from build123d import *

# Parameters (mm, degrees)
SKETCH1_R           = 1.7018
BOSS_EXTRUDE1_DEPTH = 2.5019
BOSS_EXTRUDE2_DEPTH = 4.5339
SKETCH3_R           = 2.032
BOSS_EXTRUDE3_DEPTH = 0.8128
SKETCH4_R           = 1.77918252
BOSS_EXTRUDE4_DEPTH = 1.0033


with BuildPart() as part:
    # Sketch1 → Boss-Extrude1 (new body)
    with BuildSketch(Plane(origin=(0, 0, 0), x_dir=(1, 0, 0), z_dir=(0, 1, 0))):
        with BuildLine():
            Line((27.1272, -31.8389), (27.1272, -19.9898))
            Line((27.1272, -19.9898), (25.072658108, -8.860571344))
            ThreePointArc((25.072658108, -8.860571344), (22.793680926, -7.133528849), (20.8661, -9.2456))
            Line((20.8661, -9.2456), (20.8661, -17.7038))
            ThreePointArc((20.8661, -17.7038), (21.487297228, -19.203502772), (22.987, -19.8247))
            Line((22.987, -19.8247), (23.3553, -19.8247))
            ThreePointArc((23.3553, -19.8247), (23.894115367, -20.047884633), (24.1173, -20.5867))
            Line((24.1173, -20.5867), (24.1173, -26.416))
            ThreePointArc((24.1173, -26.416), (23.496102772, -27.915702772), (21.9964, -28.5369))
            Line((21.9964, -28.5369), (11.9634, -28.5369))
            ThreePointArc((11.9634, -28.5369), (10.463697228, -27.915702772), (9.8425, -26.416))
            Line((9.8425, -26.416), (9.8425, -20.5867))
            ThreePointArc((9.8425, -20.5867), (10.065684633, -20.047884633), (10.6045, -19.8247))
            Line((10.6045, -19.8247), (10.9728, -19.8247))
            ThreePointArc((10.9728, -19.8247), (12.472502772, -19.203502772), (13.0937, -17.7038))
            Line((13.0937, -17.7038), (13.0937, -9.2456))
            ThreePointArc((13.0937, -9.2456), (11.166119074, -7.133528849), (8.887141892, -8.860571344))
            Line((8.887141892, -8.860571344), (6.8326, -19.9898))
            Line((6.8326, -19.9898), (6.8326, -31.8389))
            ThreePointArc((6.8326, -31.8389), (6.211402772, -33.338602772), (4.7117, -33.9598))
            add(Edge.make_bspline(
                [(0, -24.0873616), (0, -26.517133331), (1.36922065, -33.9598), (4.7117, -33.9598)],
                knots=[0, 0, 0, 0, 1, 1, 1, 1], degree=3))
            Line((0, -24.0873616), (0, -8.8138))
            ThreePointArc((0, -8.8138), (2.581502252, -2.581502252), (8.8138, 0))
            Line((8.8138, 0), (25.146, 0))
            ThreePointArc((25.146, 0), (31.378297748, -2.581502252), (33.9598, -8.8138))
            Line((33.9598, -8.8138), (33.9598, -24.0873616))
            add(Edge.make_bspline(
                [(33.9598, -24.0873616), (33.9598, -26.517133331), (32.59057935, -33.9598), (29.2481, -33.9598)],
                knots=[0, 0, 0, 0, 1, 1, 1, 1], degree=3))
            ThreePointArc((29.2481, -33.9598), (27.748397228, -33.338602772), (27.1272, -31.8389))
        make_face()
        with Locations((30.1117, -16.9164)):
            Circle(SKETCH1_R, mode=Mode.SUBTRACT)
        with Locations((3.8481, -16.9164)):
            Circle(SKETCH1_R, mode=Mode.SUBTRACT)
    extrude(amount=BOSS_EXTRUDE1_DEPTH)

    # Sketch2 → Boss-Extrude2 (add)
    with BuildSketch(Plane(origin=(0, 2.5019, 0), x_dir=(1, 0, 0), z_dir=(0, 1, 0))):
        Polygon((8.0899, -16.9164), (25.8699, -16.9164), (23.67915, -10.1473), (10.28065, -10.1473), align=None)
    extrude(amount=BOSS_EXTRUDE2_DEPTH)

    # Sketch3 → Boss-Extrude3 (add)
    with BuildSketch(Plane(origin=(0, 7.0358, 0), x_dir=(-1, 0, 0), z_dir=(0, 1, 0))):
        with Locations((-16.9799, 13.53185)):
            Circle(SKETCH3_R)
    extrude(amount=BOSS_EXTRUDE3_DEPTH)

    # Sketch4 → Boss-Extrude4 (add)
    with BuildSketch(Plane.XZ):
        with Locations((13.894791914, 24.167570002)):
            Circle(SKETCH4_R)
        with Locations((20.065008086, 24.167570002)):
            Circle(SKETCH4_R)
    extrude(amount=BOSS_EXTRUDE4_DEPTH)


solid = part.part
Geometry check sheet. Reference: the model listing, model coordinates, mm. A direction names the side the tool comes from. Give positions to 0.01 mm unless a question says otherwise; leave off trailing zeros. Order: outer loops, then holes, each group sorted by start corner. A loop starts at its lowest first (then second) coordinate and runs counter-clockwise, first axis right, second up.
1. Sectioned sample at B-B (x = 19.5). Record the boundary of the cut face in (y, z), then the cut area to 3 significant figures.
Completed:
outline: (-1, 22.48) - (0, 22.48) - (0, 0) - (2.5, 0) - (2.5, 10.15) - (7.04, 10.15) - (7.04, 16.92) - (2.5, 16.92) - (2.5, 28.54) - (0, 28.54) - (0, 25.85) - (-1, 25.85) - close
area: 105 mm2
2. Sectioned sample at C-C (y = 3.5). Record the boundary of the cut face in (x, z), then the cut area to 3 significant figures.
Completed:
outline: (8.09, 16.92) - (10.28, 10.15) - (23.68, 10.15) - (25.87, 16.92) - close
area: 106 mm2
3. Sectioned sample at D-D (z = 4). Record the boundary of the cut face in (x, y), then the cut area to 3 significant figures.
Completed:
outline: (1.43, 0) - (32.53, 0) - (32.53, 2.5) - (1.43, 2.5) - close
area: 77.8 mm2
4. Draft check along Z on faces 5 (the face through (26.114, 1.233, 14.503)), 6 (the face through (30.897, 1.233, 18.426)), 7 (the face through (33.96, 1, 16)), 8 (the face through (2.513, 1.233, 2.65)). Enter one of: pulls with the +Z half, pulls with the -Z half, needs draft (parallel to the pull), parting line crosses it, or undercut.
Completed:
face 5: pulls with the +Z half
face 6: undercut
face 7: needs draft
face 8: pulls with the -Z half
5. Access from +Z, -Z, +X, -X, +Y, -Y to the whole of each face (thin tool, end or side, straight path). Record for faces 1 (the face through (18.478, 7.437, 14.905)), 2 (the face through (23, 2.502, 13)), 3 (the face through (22.84, 1.23, 7.13)), 4 (the face through (6.833, 1, 26)).
Completed:
face 1: +Y
face 2: -Y
face 3: +Y, -Y
face 4: +Z, +Y, -Y
6. Depth check by flat-ended pin: pin 1 (4.5 mm diameter, centred on x = 3.85, z = 16.92, fed in from -Y); pin 2 (1.3 mm diameter, centred on y = 2, z = 27, fed in from +X); pin 3 (9.5 mm diameter, centred on x = 17, z = 24, fed in from +Y). Enter the tip coordinate at first touch or a pass-through.
Completed:
pin 1: stops at y = 0
pin 2: stops at x = 33.74
pin 3: stops at y = 2.5
7. Scan lines: line 1 (X direction, y = 1, z = 15.5); line 2 (X direction, y = 0.5, z = 14.5); line 3 (X direction, y = 2, z = 10). Record each from-to range of solid material in increasing order.
Completed:
line 1: x = 0 to 2.9, 4.79 to 7.66, 13.09 to 20.87, 26.3 to 29.17, 31.06 to 33.96
line 2: x = 0 to 7.85, 13.09 to 20.87, 26.11 to 33.96
line 3: x = 0 to 8.68, 13.09 to 20.87, 25.28 to 33.96
8. Sectioned sample at A-A (z = 21.5). Record the boundary of the cut face in (x, y), then the cut area to 3 significant figures.
Completed:
outline: (0, 0) - (6.83, 0) - (6.83, 2.5) - (0, 2.5) - close; (9.84, 0) - (24.12, 0) - (24.12, 2.5) - (9.84, 2.5) - close; (27.13, 0) - (33.96, 0) - (33.96, 2.5) - (27.13, 2.5) - close
area: 69.9 mm2
